Verification items for the finished model (mm, model axes). Round coordinates to 2 decimals unless told otherwise and drop trailing zeros. Write each loop counter-clockwise with the first axis right and the second up, starting at its lowest first coordinate (ties: lowest second). Pieces come first, ordered by that corner, then holes. Notation, with made-up numbers: M -15,-22.75 L 15,-22.75 A22 ccw 15,10.25 Z; hole C 79,-19.75 d8. An arc over 180 degrees is marked long. Answer in a Markdown table with one row per item. Add a question column.
1. Material ranges on probe 1 along Z at (x, y) = (0, -18); probe 2 along X at (y, z) = (-18, -53); probe 3 along Z at (x, y) = (33, -15.5), recorded low to high.
2. Sectioned sample at A-A on x = 0. Record the cut outline in (y, z), plus the area to 3 significant figures.
3. Go/stop test with flat-tipped pins: pin 1 Ø17.5 at (x, z) = (-23.69, -49.2) entering from +Y; pin 2 Ø1 at (y, z) = (-22, 22.5) entering from +X; pin 3 Ø4 at (x, y) = (58.5, -13.5) entering from +Z; pin 4 Ø10 at (y, z) = (-8, -50) entering from -X. Record where each tip stops, or that it passes through.
4. Draft check along X on faces 1 (the cylindrical face through (-27.16, -12.52, 8.55)), 2 (the flat face through (29, -25.4, 1)), 3 (the cylindrical face through (70.032, -9.392, 22.054)). Enter one of: pulls with the +X half, pulls with the -X half, needs draft (parallel to the pull), parting line crosses it, or undercut.
5. Sectioned sample at B-B on y = -14. Count the separate pieces of the cut face and the enclosed holes in it, plus the area to 3 significant figures.
```python
from build123d import *

# Parameters (mm, degrees)
F0_R     = 73.4225499851
F1_DEPTH = 25.4
F3_R     = 6.35
F5_DEPTH = 25.4
F6_R     = 28.4745991817
F7_DEPTH = 25.4


with BuildPart() as f1:
    # F0 (on Front) → F1 (new body)
    with BuildSketch(Plane.XZ):
        Circle(F0_R)
    extrude(amount=F1_DEPTH)

    # F3
    f3_edges = [f1.edges().sort_by_distance(p)[0] for p in [
        (-73.42255, -25.4, 0),
    ]]
    fillet(f3_edges, radius=F3_R)

    # F4 (on face) → F5 (cut)
    with BuildSketch(Plane.XZ.offset(25.4)):
        with BuildLine():
            ThreePointArc((10.828438703, 53.2833849069), (10.8892176697, 53.9458802451), (10.9095024699, 54.6108484268))
            ThreePointArc((10.9095024699, 54.6108484268), (-0.6649681817, 65.5000660965), (-10.828438703, 53.2833849069))
            ThreePointArc((-10.828438703, 53.2833849069), (0, 54.3725499851), (10.828438703, 53.2833849069))
        make_face()
        with BuildLine():
            ThreePointArc((10.828438703, 53.2833849069), (0, 54.3725499851), (-10.828438703, 53.2833849069))
            ThreePointArc((-10.828438703, 53.2833849069), (0, 43.7013459569), (10.828438703, 53.2833849069))
        make_face()
        with BuildLine():
            ThreePointArc((-48.4100489141, 24.7556328141), (-42.5101713604, 33.9007304168), (-34.9072067114, 41.6876613819))
            ThreePointArc((-34.9072067114, 41.6876613819), (-51.2258730734, 40.8512705983), (-48.4100489141, 24.7556328141))
        make_face()
        with BuildLine():
            ThreePointArc((-31.7869781145, 34.049307065), (-32.5971155871, 38.1748459137), (-34.9072067114, 41.6876613819))
            ThreePointArc((-34.9072067114, 41.6876613819), (-42.5101713604, 33.9007304168), (-48.4100489141, 24.7556328141))
            ThreePointArc((-48.4100489141, 24.7556328141), (-37.3727104759, 24.5269798299), (-31.7869781145, 34.049307065))
        make_face()
        with BuildLine():
            ThreePointArc((48.4100489141, 24.7556328141), (42.5101713604, 33.9007304168), (34.9072067114, 41.6876613819))
            ThreePointArc((34.9072067114, 41.6876613819), (34.1670880954, 27.2473435317), (48.4100489141, 24.7556328141))
        make_face()
        with BuildLine():
            ThreePointArc((53.6059830542, 34.049307065), (46.8220194331, 44.1486720622), (34.9072067114, 41.6876613819))
            ThreePointArc((34.9072067114, 41.6876613819), (42.5101713604, 33.9007304168), (48.4100489141, 24.7556328141))
            ThreePointArc((48.4100489141, 24.7556328141), (52.2188078195, 28.7255369565), (53.6059830542, 34.049307065))
        make_face()
        with BuildLine():
            ThreePointArc((-49.5379049078, -22.4136157107), (-53.009316637, -12.0990306043), (-54.3570134948, -1.299721437))
            ThreePointArc((-54.3570134948, -1.299721437), (-63.8776189051, -14.5796496747), (-49.5379049078, -22.4136157107))
        make_face()
        with BuildLine():
            ThreePointArc((-42.3321379694, -12.1520569961), (-45.9324312127, -4.0531246824), (-54.3570134948, -1.299721437))
            ThreePointArc((-54.3570134948, -1.299721437), (-53.009316637, -12.0990306043), (-49.5379049078, -22.4136157107))
            ThreePointArc((-49.5379049078, -22.4136157107), (-44.3135063658, -18.421480104), (-42.3321379694, -12.1520569961))
        make_face()
        with BuildLine():
            ThreePointArc((49.5379049078, -22.4136157107), (53.009316637, -12.0990306043), (54.3570134948, -1.299721437))
            ThreePointArc((54.3570134948, -1.299721437), (42.6056619733, -9.7244643175), (49.5379049078, -22.4136157107))
        make_face()
        with BuildLine():
            ThreePointArc((64.1511429091, -12.1520569961), (61.340572753, -4.8428477695), (54.3570134948, -1.299721437))
            ThreePointArc((54.3570134948, -1.299721437), (53.009316637, -12.0990306043), (49.5379049078, -22.4136157107))
            ThreePointArc((49.5379049078, -22.4136157107), (59.5110635472, -21.0801910696), (64.1511429091, -12.1520569961))
        make_face()
        with BuildLine():
            ThreePointArc((-13.3627081169, -52.7049544509), (-23.5913652929, -48.9879748051), (-32.8748804356, -43.3083875044))
            ThreePointArc((-32.8748804356, -43.3083875044), (-28.4282148354, -59.031796372), (-13.3627081169, -52.7049544509))
        make_face()
        with BuildLine():
            ThreePointArc((-12.7852566419, -49.2026742823), (-20.6233841848, -38.7344413752), (-32.8748804356, -43.3083875044))
            ThreePointArc((-32.8748804356, -43.3083875044), (-23.5913652929, -48.9879748051), (-13.3627081169, -52.7049544509))
            ThreePointArc((-13.3627081169, -52.7049544509), (-12.930587523, -50.9774571271), (-12.7852566419, -49.2026742823))
        make_face()
        with BuildLine():
            ThreePointArc((13.3627081169, -52.7049544509), (23.5913652929, -48.9879748051), (32.8748804356, -43.3083875044))
            ThreePointArc((32.8748804356, -43.3083875044), (18.9613033883, -39.3735521926), (13.3627081169, -52.7049544509))
        make_face()
        with BuildLine():
            ThreePointArc((34.6042615817, -49.2026742823), (34.1629920189, -46.1312993553), (32.8748804356, -43.3083875044))
            ThreePointArc((32.8748804356, -43.3083875044), (23.5913652929, -48.9879748051), (13.3627081169, -52.7049544509))
            ThreePointArc((13.3627081169, -52.7049544509), (25.4695419566, -59.9668458711), (34.6042615817, -49.2026742823))
        make_face()
    extrude(amount=-F5_DEPTH, mode=Mode.SUBTRACT)

    # F6 (on face) → F7 (cut)
    with BuildSketch(Plane(origin=(0, 0, 0), x_dir=(-1, 0, 0), z_dir=(0, 1, 0))):
        Circle(F6_R)
    extrude(amount=-F7_DEPTH, mode=Mode.SUBTRACT)


solid = f1.part
```
Geometry check:
| question | item | result |
|---|---|---|
| 1 | probe 1 | z = -73.42 to -28.47, 28.47 to 43.7, 65.52 to 73.42 |
| 1 | probe 2 | x = -50.81 to -33.92, -13.47 to 13.47, 33.92 to 50.81 |
| 1 | probe 3 | z = -65.59 to -54.9, -43.51 to 29.05, 39.05 to 65.59 |
| 2 | outline | M -25.4,-67.07 A6.35 ccw -19.05,-73.42 L 0,-73.42 L 0,-28.47 L -25.4,-28.47 Z; M -25.4,28.47 L 0,28.47 L 0,43.7 L -25.4,43.7 Z; M -25.4,65.52 L 0,65.52 L 0,73.42 L -19.05,73.42 A6.35 ccw -25.4,67.07 Z |
| 2 | area | 1,710 mm2 |
| 3 | pin 1 | passes through |
| 3 | pin 2 | stops at x = 69.43 |
| 3 | pin 3 | stops at z = 46.89 |
| 3 | pin 4 | stops at x = -58.02 |
| 4 | face 1 | undercut |
| 4 | face 2 | needs draft |
| 4 | face 3 | parting line crosses it |
| 5 | separate pieces | 1 |
| 5 | enclosed holes | 8 |
| 5 | area | 11,800 mm2 |
